For this review, take the finished solid that the model builds, in its own axes (mm). A direction names the side the tool comes from. Coordinates: 2 decimals unless noted, no trailing zeros. Write each loop counter-clockwise with the first axis right and the second up, starting at its lowest first coordinate (ties: lowest second). Pieces come first, ordered by that corner, then holes.
1) We need section A-A on y = -6.5. Write out the cut boundary in (x, z), then the cut area to 3 significant figures.
2) Insertion check: P1, Ø1.5, axis at x = 4, y = -2, coming from the -Z side; P2, Ø3, axis at x = 0, z = 0, coming from the -Y side; P3, Ø1, axis at x = 2.5, y = -6.5, coming from the +Z side. Each pin has a flat end and moves straight along its axis. Give the tip position at first contact, or say it passes through.
3) To check wall thickness, follow line 1 along Z through (x, y) = (0, -6.1); line 2 along X through (y, z) = (-4, 1); line 3 along X through (y, z) = (-11.25, -4). State the ranges of each line that lie inside material, in increasing order.
4) Mouldability with a two-part tool opening along X and no side actions: class faces 3 (the face through (0, -6, -6)), 4 (the face through (0, 0, 0)), 5 (the face through (-4.984, -10.521, -0.654)) as pulls with the +X half, pulls with the -X half, needs draft (parallel to the pull), parting line crosses it, or undercut.
5) We need section C-C on y = -10.5. Write out the cut boundary in (x, z).
6) We need section B-B on y = -0.75. Write out the cut boundary in (x, z).
7) For faces 1 (the face through (-4, -12, 4)), 2 (the face through (-0.27, -5.9, 1.22)), list the 3-axis set-ups (+Z, -Z, +X, -X, +Y, -Y) from which the entire face can be reached by the end or side of a thin tool; tool diameter is ignored.
from build123d import *

# Parameters (mm, degrees)
M3X0_5_TAPPED_HOLE2_D     = 2.5
M3X0_5_TAPPED_HOLE2_DEPTH = 4.87
M3X0_5_TAPPED_HOLE2_TIP   = 0.751075774


with BuildPart() as part:
    # Sketch2 → Revolve1 (revolve)
    with BuildSketch(Plane(origin=(0, 0, 0), x_dir=(0, 0, -1), z_dir=(1, 0, 0))):
        Polygon((-5, -12), (-6, -12), (-6, 0), (0, 0), (0, -8.373661293), (-1.5, -8.373661293), (-5.055003164, -9.000504267), align=None)
    revolve(axis=Axis((0, 88.13248411, 0), (0, -1, 0)))

    # M3x0.5 Tapped Hole2
    with Locations(Plane(origin=(0, -8.373661293, 0), x_dir=(-1, 0, 0), z_dir=(0, -1, 0))):
        with Locations((0, 0)):
            Hole(M3X0_5_TAPPED_HOLE2_D / 2, depth=M3X0_5_TAPPED_HOLE2_DEPTH)
            with Locations((0, 0, -(M3X0_5_TAPPED_HOLE2_DEPTH + M3X0_5_TAPPED_HOLE2_TIP / 2))):  # 118° drill point
                Cone(0, M3X0_5_TAPPED_HOLE2_D / 2, M3X0_5_TAPPED_HOLE2_TIP, mode=Mode.SUBTRACT)


solid = part.part
Result:
1. outline: circle Ø12 at (0, 0); hole circle Ø2.5 at (0, 0)
1. area: 108 mm2
2. P1: stops at z = -5.04
2. P2: stops at y = -8.37
2. P3: stops at z = 5.66
3. line 1: z = -6 to -1.25, 1.25 to 6
3. line 2: x = -5.92 to -0.75, 0.75 to 5.92
3. line 3: x = -4.47 to -3.02, 3.02 to 4.47
4. face 3: parting line crosses it
4. face 4: needs draft
4. face 5: undercut
5. outline: circle Ø12 at (0, 0); hole circle Ø10.06 at (0, 0)
6. outline: circle Ø12 at (0, 0)
7. face 1: +Z, -Z, +X, -X, -Y
7. face 2: -Y
